```python
from build123d import *

# Parameters (mm, degrees)
SKETCH1_R           = 8
BOSS_EXTRUDE1_DEPTH = 12
SKETCH3_W           = 35
SKETCH3_H           = 5
CUT_EXTRUDE1_DEPTH  = 30
SKETCH4_W           = 20
SKETCH4_H           = 50
BOSS_EXTRUDE2_DEPTH = 12
FILLET1_R           = 10
FILLET2_R           = 10
SKETCH7_R           = 8.5
CUT_EXTRUDE4_DEPTH  = 12
SKETCH8_R           = 22.712934263
CUT_EXTRUDE5_DEPTH  = 4
CUT_EXTRUDE6_START  = -4
SKETCH9_R           = 22.712934263
CUT_EXTRUDE6_DEPTH  = 4
SKETCH14_R          = 2.25
CUT_EXTRUDE7_DEPTH  = 12
FILLET3_R           = 5
FILLET4_R           = 5
SKETCH15_R          = 8.5
CUT_EXTRUDE8_DEPTH  = 12
CUT_EXTRUDE9_DEPTH  = 7
CHAMFER1_START      = 3.5
CHAMFER1_DEPTH      = 5
FILLET6_R           = 7
FILLET7_R           = 7
FILLET9_R           = 2
FILLET10_R          = 2


with BuildPart() as part:
    # Sketch1 → Boss-Extrude1 (new body)
    with BuildSketch(Plane(origin=(0, 0, 0), x_dir=(1, 0, 0), z_dir=(0, 1, 0))):
        with BuildLine():
            Line((0, 15), (130, 15))
            ThreePointArc((130, 15), (145, 0), (130, -15))
            Line((130, -15), (0, -15))
            ThreePointArc((0, -15), (-15, 0), (0, 15))
        make_face()
        with Locations(Location((0, 0, 0), (0, 0, 270))):
            Circle(SKETCH1_R, mode=Mode.SUBTRACT)
    extrude(amount=BOSS_EXTRUDE1_DEPTH)

    # Sketch3 → Cut-Extrude1 (cut)
    with BuildSketch(Plane(origin=(0, 0, -15), x_dir=(-1, 0, 0), z_dir=(0, 0, -1))):
        with Locations((-2.5, 6)):
            Rectangle(SKETCH3_W, SKETCH3_H)
    extrude(amount=-CUT_EXTRUDE1_DEPTH, mode=Mode.SUBTRACT)

    # Sketch4 → Boss-Extrude2 (add)
    with BuildSketch(Plane.XZ):
        with Locations((120, -40)):
            Rectangle(SKETCH4_W, SKETCH4_H)
    extrude(amount=-BOSS_EXTRUDE2_DEPTH)

    # Fillet1
    fillet1_edges = [part.edges().sort_by_distance(p)[0] for p in [
        (110, 6, -65),
    ]]
    fillet(fillet1_edges, radius=FILLET1_R)

    # Fillet2
    fillet2_edges = [part.edges().sort_by_distance(p)[0] for p in [
        (130, 6, -65),
    ]]
    fillet(fillet2_edges, radius=FILLET2_R - 0.0001)  # a hair under: the kernel refuses the full size

    # Sketch7 → Cut-Extrude4 (cut)
    with BuildSketch(Plane.XZ):
        with Locations(Location((130, 0, 0), (0, 0, 270))):
            Circle(SKETCH7_R)
    extrude(amount=-CUT_EXTRUDE4_DEPTH, mode=Mode.SUBTRACT)

    # Sketch8 → Cut-Extrude5 (cut)
    with BuildSketch(Plane(origin=(0, 12, 0), x_dir=(1, 0, 0), z_dir=(0, 1, 0))):
        with Locations((133.938996952, -3.822545113)):
            Circle(SKETCH8_R)
    extrude(amount=-CUT_EXTRUDE5_DEPTH, mode=Mode.SUBTRACT)

    # Sketch9 → Cut-Extrude6 (cut)
    with BuildSketch(Plane.XZ.offset(CUT_EXTRUDE6_START)):
        with Locations((133.938996952, 3.822545113)):
            Circle(SKETCH9_R)
    extrude(amount=CUT_EXTRUDE6_DEPTH, mode=Mode.SUBTRACT)

    # Sketch14 → Cut-Extrude7 (cut)
    with BuildSketch(Plane.XZ):
        with Locations(Location((116.3, -53, 0), (0, 0, 270))):
            Circle(SKETCH14_R)
        with Locations(Location((123.8, -53, 0), (0, 0, 270))):
            Circle(SKETCH14_R)
    extrude(amount=-CUT_EXTRUDE7_DEPTH, mode=Mode.SUBTRACT)

    # Fillet3
    fillet3_edges = [part.edges().sort_by_distance(p)[0] for p in [
        (114.166746572, 10, 15),
    ]]
    fillet(fillet3_edges, radius=FILLET3_R)

    # Fillet4
    fillet4_edges = [part.edges().sort_by_distance(p)[0] for p in [
        (114.166746572, 2, 15),
    ]]
    fillet(fillet4_edges, radius=FILLET4_R)

    # Sketch15 → Cut-Extrude8 (cut)
    with BuildSketch(Plane.XZ):
        with Locations(Location((37.060545973, 4.039960241, 0), (0, 0, 270))):
            Circle(SKETCH15_R)
    extrude(amount=-CUT_EXTRUDE8_DEPTH, mode=Mode.SUBTRACT)

    # Sketch16 → Cut-Extrude9 (cut)
    with BuildSketch(Plane.XY.offset(15)):
        with BuildLine():
            Line((60.046424392, 3.5), (30.046424392, 3.5))
            ThreePointArc((30.046424392, 3.5), (27.546424392, 6), (30.046424392, 8.5))
            Line((30.046424392, 8.5), (60.046424392, 8.5))
            ThreePointArc((60.046424392, 8.5), (62.546424392, 6), (60.046424392, 3.5))
        make_face()
    extrude(amount=-CUT_EXTRUDE9_DEPTH, mode=Mode.SUBTRACT)

    # Chamfer1: read off the stored shape, not the designer's step
    # Chamfer1 outline → Chamfer1 (cut)
    with BuildSketch(Plane(origin=(0, 0, 0), x_dir=(1, 0, 0), z_dir=(0, 1, 0)).offset(CHAMFER1_START)):
        with BuildLine():
            Line((44.581721752, -8), (54.625922679, -8))
            Line((54.625922679, -8), (45.554566675, -3.721193369))
            ThreePointArc((45.554566675, -3.721193369), (45.349012425, -5.924455895), (44.581721752, -8))
        make_face()
    extrude(amount=CHAMFER1_DEPTH, mode=Mode.SUBTRACT)

    # Fillet6
    fillet6_edges = [part.edges().sort_by_distance(p)[0] for p in [
        (130, 2, -18.546220742),
    ]]
    fillet(fillet6_edges, radius=FILLET6_R)

    # Fillet7
    fillet7_edges = [part.edges().sort_by_distance(p)[0] for p in [
        (130, 10, -18.546220742),
    ]]
    fillet(fillet7_edges, radius=FILLET7_R)

    # Fillet9
    fillet9_edges = [part.edges().sort_by_distance(p)[0] for p in [
        (20, 6, -15),
    ]]
    fillet(fillet9_edges, radius=FILLET9_R)

    # Fillet10
    fillet10_edges = [part.edges().sort_by_distance(p)[0] for p in [
        (20, 6, 15),
    ]]
    fillet(fillet10_edges, radius=FILLET10_R)


solid = part.part
```
Geometry check sheet. Reference: the model listing, model coordinates, mm. A direction names the side the tool comes from. Give positions to 0.01 mm unless a question says otherwise; leave off trailing zeros. Order: outer loops, then holes, each group sorted by start corner. A loop starts at its lowest first (then second) coordinate and runs counter-clockwise, first axis right, second up.
1. Release check for a two-part mould opening along Y. For faces 6 (the face through (68, 12, -7)), 7 (the face through (-15, 10, 0)), 8 (the face through (49, 3.5, 12)) record: pulls with the +Y half, pulls with the -Y half, needs draft (parallel to the pull), parting line crosses it, or undercut.
2. Thickness scan on L1, parallel to X at y = 5.25, z = -53; L2, parallel to X at y = 9.5, z = -51; L3, parallel to Y at x = 7, z = -14.5. Record the ranges inside material, lowest first.
3. Section check B-B, the plane x = 116.3. Enter the section's corners in (y, z).
4. Section check A-A, the plane z = -53. Enter the section's corners in (x, y).
5. Section check D-D, the plane y = 5.75. Give the number of separate pieces and of enclosed holes in the cut face, and give its area (3 significant figures).
6. Section check C-C, the plane z = 0. Enter the section's corners in (x, y), and give its area (3 significant figures).
7. Access from +Z, -Z, +X, -X, +Y, -Y to the whole of each face (thin tool, end or side, straight path). Record for faces 1 (the face through (62.546, 6.055, 11.549)), 2 (the face through (128.757, 2.028, -19.821)), 3 (the face through (110, 6, -35)), 4 (the face through (-15, 2, 0)), 5 (the face through (128.757, 10.028, -19.821)).
8. Gauge pin test, flat ends, axial feed: pin 1 Ø1.5 at (y, z) = (5, 5.5) entering from -X; pin 2 Ø6 at (y, z) = (4, -33.5) entering from -X; pin 3 Ø2.5 at (x, y) = (57, 6) entering from +Z. Record the tip position at first contact, or that the pin passes through.
Values follow:
1. face 6: pulls with the +Y half
1. face 7: needs draft
1. face 8: undercut
2. L1: x = 110 to 114.05, 118.55 to 121.55, 126.05 to 130
2. L2: x = 110 to 115.27, 117.33 to 122.77, 124.83 to 130
2. L3: y = 0 to 3.5, 8.5 to 12
3. outline: (0, -64.29) - (12, -64.29) - (12, -55.25) - (0, -55.25) - close; (0, -50.75) - (12, -50.75) - (12, -10.49) - (8, -10.49) - (8, 15) - (4, 15) - (4, -10.49) - (0, -10.49) - close
4. outline: (110, 0) - (114.05, 0) - (114.05, 12) - (110, 12) - close; (118.55, 0) - (121.55, 0) - (121.55, 12) - (118.55, 12) - close; (126.05, 0) - (130, 0) - (130, 12) - (126.05, 12) - close
5. separate pieces: 1
5. enclosed holes: 3
5. area: 3,910 mm2
6. outline: (-15, 0) - (-8, 0) - (-8, 3.5) - (-15, 3.5) - close; (-15, 8.5) - (-8, 8.5) - (-8, 12) - (-15, 12) - close; (8, 0) - (29.58, 0) - (29.58, 12) - (8, 12) - (8, 8.5) - (20, 8.5) - (20, 3.5) - (8, 3.5) - close; (44.54, 0) - (111.55, 0) - (111.55, 4) - (121.5, 4) - (121.5, 8) - (111.55, 8) - (111.55, 12) - (44.54, 12) - close; (138.5, 4) - (145, 4) - (145, 8) - (138.5, 8) - close
6. area: 1,120 mm2
7. face 1: +Z
7. face 2: +Z, +X, -Y
7. face 3: -Z, -X, +Y, -Y
7. face 4: -X, +Y, -Y
7. face 5: +Z, +X, +Y
8. pin 1: stops at x = 20
8. pin 2: stops at x = 110
8. pin 3: stops at z = 8
